Job drawing, mm, ordinate dimensions from the low corner. One solid piece. Give positions to 0.01 mm unless a question says otherwise; leave off trailing zeros. Order: outer loops, then holes, each group sorted by start corner. A loop starts at its lowest first (then second) coordinate and runs counter-clockwise, first axis right, second up. Notation, with made-up numbers: (13.25, 23) -> (29.25, 23) arc R23 ccw to (29.25, 61) -> close; hole circle Ø10 at (-28.5, 33). An arc over 180 degrees is marked (long way). Write item = value, one per line. Start each with the question number.
(1) Flat gauge pins, fed straight in: pin 1 (7 mm diameter, centred on x = 5.75, y = 65.75, fed in from +Z); pin 2 (5 mm diameter, centred on x = 25.5, z = 6, fed in from -Y); pin 3 (14.5 mm diameter, centred on x = 47.5, y = 17.5, fed in from +Z); pin 4 (2 mm diameter, centred on y = 42, z = 3.5, fed in from -X). Where does each tip first touch, or does it go through?
(2) Probe line 1 along X through (y, z) = (65.75, 7.25); line 2 along X through (y, z) = (7, 3.5) (1 decimal). List the from-to ranges inside material, lowest first. Write a range as from..to.
(3) Saw through at D-D, the plane y = 59. List the corners of the cut face in (x, z).
(4) Saw through at B-B, the plane z = 1. List the corners of the cut face in (x, y).
(5) Saw through at C-C, the plane x = 65.75. List the corners of the cut face in (y, z).
(6) Two-plate mould, pull along Y, no slides. Class the marked faces 1 and 2: pulls with the +Y half, pulls with the -Y half, needs draft (parallel to the pull), parting line crosses it, or undercut.
(7) Saw through at A-A, the plane z = 9. List the corners of the cut face in (x, y), then the cut area to 3 significant figures.
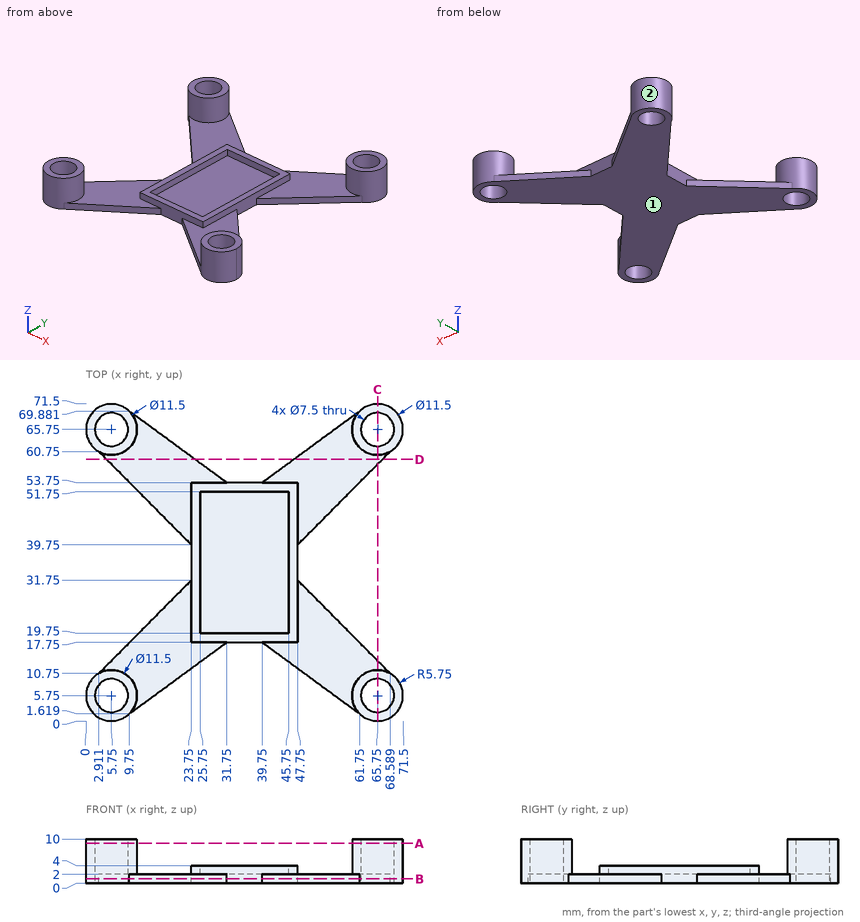
Results list:
q1.pin_1 = through
q1.pin_2 = 17.75
q1.pin_3 = 4
q1.pin_4 = 23.75
q2.line_1 = 0..2, 9.5..11.5, 60..62, 69.5..71.5
q2.line_2 = 0.1..2.2, 9.3..11.4, 60.1..62.2, 69.3..71.4
q3.outline = (4.65, 0) -> (24.59, 0) -> (24.59, 2) -> (4.65, 2) -> close; (46.91, 0) -> (66.85, 0) -> (66.85, 2) -> (46.91, 2) -> close
q4.outline = (2.91, 10.75) arc R5.75 ccw (long way) to (9.75, 1.62) -> (31.75, 17.75) -> (39.75, 17.75) -> (61.75, 1.62) arc R5.75 ccw (long way) to (68.59, 10.75) -> (47.75, 31.75) -> (47.75, 39.75) -> (68.59, 60.75) arc R5.75 ccw (long way) to (61.75, 69.88) -> (39.75, 53.75) -> (31.75, 53.75) -> (9.75, 69.88) arc R5.75 ccw (long way) to (2.91, 60.75) -> (23.75, 39.75) -> (23.75, 31.75) -> close; hole circle Ø7.5 at (5.75, 5.75); hole circle Ø7.5 at (5.75, 65.75); hole circle Ø7.5 at (65.75, 5.75); hole circle Ø7.5 at (65.75, 65.75)
q5.outline = (0, 0) -> (2, 0) -> (2, 10) -> (0, 10) -> close; (9.5, 0) -> (13.61, 0) -> (13.61, 2) -> (11.5, 2) -> (11.5, 10) -> (9.5, 10) -> close; (57.89, 0) -> (62, 0) -> (62, 10) -> (60, 10) -> (60, 2) -> (57.89, 2) -> close; (69.5, 0) -> (71.5, 0) -> (71.5, 10) -> (69.5, 10) -> close
q6.face_1 = needs draft
q6.face_2 = undercut
q7.outline = circle Ø11.5 at (5.75, 5.75); circle Ø11.5 at (5.75, 65.75); circle Ø11.5 at (65.75, 5.75); circle Ø11.5 at (65.75, 65.75); hole circle Ø7.5 at (5.75, 5.75); hole circle Ø7.5 at (5.75, 65.75); hole circle Ø7.5 at (65.75, 5.75); hole circle Ø7.5 at (65.75, 65.75)
q7.area = 239 mm^2
